Check sheet for the modelled part. Datum: model origin and axes. Units: mm. A direction names the side the tool comes from. Give positions to 0.01 mm unless a question says otherwise; leave off trailing zeros. Write each loop counter-clockwise with the first axis right and the second up, starting at its lowest first coordinate (ties: lowest second). Pieces come first, ordered by that corner, then holes. Notation, with made-up numbers: M 0,-32 L 20,-32 A25 cw 20,-4 Z; hole C 37.5,-23.75 d11. An arc over 180 degrees is marked long. Write item = value, one per line. Start each with the question number.
1) Cross-section at D-D, the plane y = -9. Give the number of separate pieces and of enclosed holes in the cut face, plus the area to 3 significant figures.
2) Access from +Z, -Z, +X, -X, +Y, -Y to the whole of each face (thin tool, end or side, straight path). Record for faces 5 (the flat face through (-5.5, -6.26, 43.65)), 6 (the flat face through (10.56, -6.26, 35.32)), 7 (the flat face through (-10.613, -6.261, 14.022)).
3) Go/stop test with flat-tipped pins: pin 1 (6.5 mm diameter, centred on x = 47.5, y = -5.5, fed in from +Z); pin 2 (2 mm diameter, centred on x = 4.5, y = -8.5, fed in from -Z); pin 3 (0.8 mm diameter, centred on x = 1.5, y = -6, fed in from +Z). Record where each tip stops, or that it passes through.
4) Cross-section at A-A, the plane z = -45. Record the cut outline in (x, y).
5) Mould release check, pull along X, two halves, no side actions. Record for faces 1 (the flat face through (-4.614, -6.261, 22.448)), 2 (the flat face through (7.22, -6.26, 17.92)), 3 (the flat face through (-9.606, -6.261, 19.916)), 4 (the flat face through (0.975, -6, 84)): released by +X, released by -X, zero draft, split by the parting line, or undercut.
6) Cross-section at B-B, the plane x = -31. Record the cut outline in (y, z), plus the area to 3 significant figures.
7) Scan lines: line 1 along X through (y, z) = (-6.5, 15.5); line 2 along X through (y, z) = (-8.75, -43.5); line 3 along Z through (x, y) = (9, -7.75). Record each from-to range of solid material in increasing order. Write a range as [from, to].
8) Cross-section at C-C, the plane x = -47. Record the cut outline in (y, z), plus the area to 3 significant figures.
```python
from build123d import *

# Parameters (mm, degrees)
F0_R     = 0.453147
F0_R_2   = 0.54441
F0_R_3   = 0.54854
F1_DEPTH = 12.7


with BuildPart() as f1:
    # F0 (on Front) → F1 (new body)
    with BuildSketch(Plane.XZ):
        Polygon((-39.533757, -65.54234), (-0.760193, -36.696203), (35.802592, -63.547), (38.606675, -65.606249), (31.076437, -42.409137), (24.738393, -22.884612), (23.723046, -19.756807), (46.13781, -3.457308), (60.679827, 7.501139), (61.14725, 8.591791), (11.964072, 8.591791), (10.218171, 17.820274), (9.674744, 25.812406), (8.968875, 25.819117), (7.777616, 30.226135), (7.229322, 32.704141), (13.991971, 38.017649), (13.720257, 43.180205), (17.780535, 43.698543), (17.675199, 44.568963), (17.675199, 44.719916), (8.1342, 54.03503), (4.368194, 59.564289), (5.838566, 63.279467), (4.368194, 69.924787), (1.731881, 79.677723), (1.555634, 81.05831), (1.212185, 81.745215), (2.003027, 82.140632), (2.027594, 82.16323), (2.027594, 82.605079), (0.975498, 82.605079), (0.975498, 85.611068), (0, 85.967864), (-0.211868, 85.971788), (-0.211868, 85.986815), (-0.452347, 86.242326), (-0.571582, 87.859698), (-0.888215, 87.865561), (-0.918275, 86.242326), (-1.534503, 85.415684), (-2.044514, 83.477632), (-1.534503, 82.935743), (-2.917258, 82.18424), (-3.007438, 81.703283), (-2.507543, 81.552982), (-2.507543, 81.424944), (-1.669773, 80.230348), (-1.669773, 80.004901), (-0.512467, 74.774474), (0, 70.505977), (0.239031, 67.845672), (-0.250665, 66.842255), (-0.873186, 68.071127), (-0.918276, 68.236455), (-1.669773, 70.175312), (-3.007438, 71.197353), (-4.765941, 71.197353), (-4.877486, 71.194044), (-5.998397, 70.626214), (-6.479356, 69.333635), (-6.479356, 69.19837), (-5.592589, 65.155312), (-4.435283, 62.870763), (-5.592589, 62.059145), (-5.592589, 61.938908), (-5.592589, 60.94693), (-6.419236, 60.105253), (-6.479356, 60.045134), (-6.479356, 59.023097), (-7.306002, 55.92693), (-6.569892, 51.117349), (-4.931271, 45.691539), (-6.079414, 41.555599), (-5.472349, 40.611416), (-6.885163, 36.538303), (-7.561511, 30.826923), (-9.079536, 23.672668), (-10.146662, 16.052486), (-11.093548, 11.934282), (-14.841024, 9.524833), (-14.841024, 8.591791), (-62.628269, 7.850908), (-25.927428, -19.620989), align=None)
        with Locations((-1.263964, 54.393876)):
            Circle(F0_R, mode=Mode.SUBTRACT)
        with Locations((-2.015462, 57.475016)):
            Circle(F0_R_2, mode=Mode.SUBTRACT)
        with Locations((-2.60163, 60.420882)):
            Circle(F0_R_3, mode=Mode.SUBTRACT)
        Polygon((6.005918, 9.801562), (6.005918, 8.591791), (-6.569892, 8.591791), (-6.723631, 13.368296), (-6.477118, 13.368296), (-5.239312, 18.816557), (-3.971315, 26.183013), (0.678006, 33.549469), (4.451805, 26.152823), (4.542376, 26.092442), (5.115994, 25.458444), (6.759554, 20.360412), (7.697042, 15.405042), (7.697042, 11.400443), align=None, mode=Mode.SUBTRACT)
    extrude(amount=F1_DEPTH)


solid = f1.part
```
Reply:
q1.separate_pieces = 1
q1.enclosed_holes = 4
q1.area = 5,140 mm2
q2.face_5 = -X, +Y, -Y
q2.face_6 = +X, +Y, -Y
q2.face_7 = +Z, -X, +Y, -Y
q3.pin_1 = 8.59
q3.pin_2 = -41.29
q3.pin_3 = 82.61
q4.outline = M -33.45,-12.7 L -11.92,-12.7 L -11.92,0 L -33.45,0 Z; M 10.55,-12.7 L 31.92,-12.7 L 31.92,0 L 10.55,0 Z
q5.face_1 = undercut
q5.face_2 = undercut
q5.face_3 = released by -X
q5.face_4 = released by +X
q6.outline = M -12.7,-59.19 L 0,-59.19 L 0,-36.74 L -12.7,-36.74 Z; M -12.7,-15.82 L 0,-15.82 L 0,8.34 L -12.7,8.34 Z
q6.area = 592 mm2
q7.line_1 = [-10.27, -5.99], [7.68, 10.66]
q7.line_2 = [-33, -9.91], [8.5, 31.43]
q7.line_3 = [-43.86, 25.82], [34.1, 53.19]
q8.outline = M -12.7,-3.85 L 0,-3.85 L 0,8.09 L -12.7,8.09 Z
q8.area = 152 mm2
